```python
from build123d import *

# Parameters (mm, degrees)
SKETCH1_R           = 6.35
BOSS_EXTRUDE1_DEPTH = 58.42
BOSS_EXTRUDE3_START = -2.54
SKETCH7_W           = 10.16
SKETCH7_H           = 2.54
BOSS_EXTRUDE3_DEPTH = 27.94
SKETCH10_R          = 1.55
CUT_EXTRUDE2_DEPTH  = 64.384429767
SKETCH13_R          = 4.826
CUT_EXTRUDE3_DEPTH  = 72.389091006


# Read off the part's stored shape, not the designer's step: Boss-Extrude2, Boss-Extrude4
with BuildPart() as part:
    # Sketch1 → Boss-Extrude1 (new body)
    with BuildSketch(Plane.XY):
        with Locations(Location((0, 0, 0), (0, 0, 180))):
            Circle(SKETCH1_R)
    extrude(amount=BOSS_EXTRUDE1_DEPTH)

    # Boss-Extrude2 outline → Boss-Extrude2 (revolve)
    with BuildSketch(Plane.XY.offset(19.812)):
        Polygon((6.35, -13.97), (6.35, -6.35), (6.257921095, -1.074803042), (0, -1.074803042), (0, -13.97), align=None)
    revolve(axis=Axis((0, 0, 19.812), (0, 1, 0)))

    # Sketch7 → Boss-Extrude3 (add)
    with BuildSketch(Plane(origin=(6.211237265, 1.320239237, 0), x_dir=(0.20791169081776328, -0.9781476007338049, 0), z_dir=(0.9781476007338049, 0.20791169081776328, 0)).offset(BOSS_EXTRUDE3_START)):
        with Locations((0, -51.562)):
            Rectangle(SKETCH7_W, SKETCH7_H)
    extrude(amount=BOSS_EXTRUDE3_DEPTH)

    # Sketch10 → Cut-Extrude2 (cut, through all)
    with BuildSketch(Plane.XY.offset(52.832)):
        with Locations((23.602701606, 5.016909099)):
            Circle(SKETCH10_R)
    extrude(amount=-CUT_EXTRUDE2_DEPTH, mode=Mode.SUBTRACT)

    # Boss-Extrude4 outline → Boss-Extrude4 (revolve)
    with BuildSketch(Plane.XY.offset(19.812)):
        Polygon((0, 6.350021501), (0, 1.075341111), (6.257930487, 1.075341111), (6.350000375, 6.350021501), align=None)
    revolve(axis=Axis((0, 0, 19.812), (0, 1, 0)))

    # Sketch13 → Cut-Extrude3 (cut, through all)
    with BuildSketch(Plane.XZ.offset(13.97)):
        with Locations(Location((0, 19.812, 0), (0, 0, 270))):
            Circle(SKETCH13_R)
    extrude(amount=-CUT_EXTRUDE3_DEPTH, mode=Mode.SUBTRACT)


solid = part.part
```
Could you check a few things on this model? Use its own coordinates, in mm. A direction names the side the tool comes from. Round coordinates to 2 decimals unless told otherwise and drop trailing zeros. Loops run counter-clockwise (first coordinate to the right, second up) from the corner with the lowest first, then second, coordinate; pieces in that order, holes last.
Q1. Thinking about a two-plate mould opening in X: for faces 6 (the flat face through (18.256, -1.313, 51.58)), 7 (the conical face through (-6.31, -4.26, 19.67)), 8 (the cylindrical face through (-1.848, -3.952, 15.354)), 9 (the cylindrical face through (22.054, 5.085, 51.58)), which applies, pulls with the +X half, pulls with the -X half, needs draft (parallel to the pull), parting line crosses it, or undercut?
Q2. On a 3-axis mill with a long thin cutter (end or side, diameter ignored), from which of +Z, -Z, +X, -X, +Y, -Y can I reach the whole of each face in a straight line? I mean faces 1 (the flat face through (0, 0, 0)), 2 (the flat face through (5, -13.97, 18)), 3 (the conical face through (6.312, -4.263, 19.951)), 4 (the cylindrical face through (-0.827, -10.107, 13.516)), 5 (the conical face through (-4.662, 4.922, 15.537)). Say none if no direction works.
Q3. I want a section at A-A (y = 0). Write out the boundary of the cut face in (x, z).
Q4. I want a section at D-D (y = -8.75). Write out the boundary of the cut face in (x, z), and give its area (3 significant figures).
Q5. I want a section at C-C (x = 20). Write out the boundary of the cut face in (y, z), and give its area (3 significant figures).
Q6. For P1, Ø1.9, axis at x = 23.6, y = 5.02, coming from the +Z side; P2, Ø10, axis at x = 0.5, z = 21, coming from the +Y side; P3, Ø4.5, axis at x = 13.5, y = 6, coming from the -Z side; P4, Ø12, axis at x = 22.5, y = 3.5, coming from the +Z side, each with a flat end and sliding along its axis, tell me the tip position at first contact or that it passes through.
Q7. I want a section at B-B (z = 45). Write out the boundary of the cut face in (x, y), and give its area (3 significant figures).
Q8. Please list where these lines run through material, in increasing order: L1, parallel to Y at x = -3, z = 15; L2, parallel to Z at x = 18.5, y = -0.5; L3, parallel to X at y = -4, z = 20.
Answer below:
1. face 6: pulls with the +X half
1. face 7: pulls with the -X half
1. face 8: undercut
1. face 9: undercut
2. face 1: -Z, +X, -X, +Y, -Y
2. face 2: +Z, -Z, +X, -X, -Y
2. face 3: +X
2. face 4: -Y
2. face 5: none
3. outline: (-6.35, 0) - (6.35, 0) - (6.35, 50.29) - (24.43, 50.29) - (24.43, 52.83) - (6.35, 52.83) - (6.35, 58.42) - (-6.35, 58.42) - close; hole circle Ø9.65 at (0, 19.81)
4. outline: circle Ø12.7 at (0, 19.81); hole circle Ø9.65 at (0, 19.81)
4. area: 53.5 mm2
5. outline: (-0.94, 50.29) - (9.44, 50.29) - (9.44, 52.83) - (-0.94, 52.83) - close
5. area: 26.4 mm2
6. P1: passes through
6. P2: stops at y = 6.35
6. P3: stops at z = 50.29
6. P4: stops at z = 52.83
7. outline: circle Ø12.7 at (0, 0)
7. area: 127 mm2
8. L1: y = -13.97 to 6.35
8. L2: z = 50.29 to 52.83
8. L3: x = -6.31 to -4.82, 4.82 to 6.31
